from build123d import *

# Parameters (mm, degrees)
SKETCH1_W             = 80
SKETCH1_H             = 225
BOSS_EXTRUDE1_DEPTH   = 29
CUT_EXTRUDE1_REACH    = 124.871
SKETCH3_R             = 8
CUT_EXTRUDE2_DEPTH    = 20
M8_TAPPED_HOLE1_D     = 6.8
M8_TAPPED_HOLE1_DEPTH = 19.75
M8_TAPPED_HOLE1_TIP   = 2.042926105
CUT_EXTRUDE3_REACH    = 124.871
SKETCH15_W            = 12
SKETCH15_H            = 11.5
SKETCH16_R            = 8.5
CUT_EXTRUDE4_DEPTH    = 5
CUT_EXTRUDE5_REACH    = 124.871
SKETCH17_R            = 4


with BuildPart() as part:
    # Sketch1 → Boss-Extrude1 (new body)
    with BuildSketch(Plane(origin=(0, 0, 0), x_dir=(1, 0, 0), z_dir=(0, 1, 0))):
        Rectangle(SKETCH1_W, SKETCH1_H)
    extrude(amount=-BOSS_EXTRUDE1_DEPTH)

    # Sketch2 → Cut-Extrude1 (cut, up to next)
    with BuildSketch(Plane(origin=(0, 0, 0), x_dir=(1, 0, 0), z_dir=(0, 1, 0)), mode=Mode.PRIVATE) as cut_extrude1_sk1:
        with BuildLine():
            Line((30.5, 72.87), (30.5, 95.77))
            ThreePointArc((30.5, 95.77), (33, 98.27), (35.5, 95.77))
            Line((35.5, 95.77), (35.5, 72.87))
            ThreePointArc((35.5, 72.87), (33, 70.37), (30.5, 72.87))
        make_face()
    cut_extrude1_tool1 = extrude(cut_extrude1_sk1.sketch, amount=-CUT_EXTRUDE1_REACH, mode=Mode.PRIVATE) & part.part
    # Sketch2 → Cut-Extrude1 (cut, up to next)
    with BuildSketch(Plane(origin=(0, 0, 0), x_dir=(1, 0, 0), z_dir=(0, 1, 0)), mode=Mode.PRIVATE) as cut_extrude1_sk2:
        with BuildLine():
            Line((30.5, 33.86), (30.5, 48.36))
            ThreePointArc((30.5, 48.36), (33, 50.86), (35.5, 48.36))
            Line((35.5, 48.36), (35.5, 33.86))
            ThreePointArc((35.5, 33.86), (33, 31.36), (30.5, 33.86))
        make_face()
    cut_extrude1_tool2 = extrude(cut_extrude1_sk2.sketch, amount=-CUT_EXTRUDE1_REACH, mode=Mode.PRIVATE) & part.part
    # Sketch2 → Cut-Extrude1 (cut, up to next)
    with BuildSketch(Plane(origin=(0, 0, 0), x_dir=(1, 0, 0), z_dir=(0, 1, 0)), mode=Mode.PRIVATE) as cut_extrude1_sk3:
        with BuildLine():
            Line((31.5, -47.14), (31.5, -18.14))
            ThreePointArc((31.5, -18.14), (31.207106781, -17.432893219), (30.5, -17.14))
            Line((30.5, -17.14), (-7.5, -17.14))
            ThreePointArc((-7.5, -17.14), (-8.207106781, -17.432893219), (-8.5, -18.14))
            Line((-8.5, -18.14), (-8.5, -47.14))
            ThreePointArc((-8.5, -47.14), (-7.035533906, -50.675533906), (-3.5, -52.14))
            Line((-3.5, -52.14), (26.5, -52.14))
            ThreePointArc((26.5, -52.14), (30.035533906, -50.675533906), (31.5, -47.14))
        make_face()
    cut_extrude1_tool3 = extrude(cut_extrude1_sk3.sketch, amount=-CUT_EXTRUDE1_REACH, mode=Mode.PRIVATE) & part.part
    # Sketch2 → Cut-Extrude1 (cut, up to next)
    with BuildSketch(Plane(origin=(0, 0, 0), x_dir=(1, 0, 0), z_dir=(0, 1, 0)), mode=Mode.PRIVATE) as cut_extrude1_sk4:
        with BuildLine():
            Line((30.5, -95.77), (30.5, -72.87))
            ThreePointArc((30.5, -72.87), (33, -70.37), (35.5, -72.87))
            Line((35.5, -72.87), (35.5, -95.77))
            ThreePointArc((35.5, -95.77), (33, -98.27), (30.5, -95.77))
        make_face()
    cut_extrude1_tool4 = extrude(cut_extrude1_sk4.sketch, amount=-CUT_EXTRUDE1_REACH, mode=Mode.PRIVATE) & part.part
    add(cut_extrude1_tool1.solids().sort_by_distance((33, 0, -84.32))[0], mode=Mode.SUBTRACT)
    add(cut_extrude1_tool2.solids().sort_by_distance((33, 0, -41.11))[0], mode=Mode.SUBTRACT)
    add(cut_extrude1_tool3.solids().sort_by_distance((11.5, 0, 34.518764))[0], mode=Mode.SUBTRACT)
    add(cut_extrude1_tool4.solids().sort_by_distance((33, 0, 84.32))[0], mode=Mode.SUBTRACT)

    # Sketch3 → Cut-Extrude2 (cut)
    with BuildSketch(Plane(origin=(0, 0, 0), x_dir=(1, 0, 0), z_dir=(0, 1, 0))):
        with Locations(Location((15, 72.5, 0), (0, 0, 270))):
            Circle(SKETCH3_R)
        with Locations(Location((15, 41.11, 0), (0, 0, 270))):
            Circle(SKETCH3_R)
        with Locations(Location((15, -7, 0), (0, 0, 270))):
            Circle(SKETCH3_R)
        with Locations(Location((15, -72.5, 0), (0, 0, 270))):
            Circle(SKETCH3_R)
        with Locations(Location((-20, -72.5, 0), (0, 0, 270))):
            Circle(SKETCH3_R)
        with Locations(Location((-20, -7, 0), (0, 0, 270))):
            Circle(SKETCH3_R)
        with Locations(Location((-20, 41.11, 0), (0, 0, 270))):
            Circle(SKETCH3_R)
        with Locations(Location((-20, 72.5, 0), (0, 0, 270))):
            Circle(SKETCH3_R)
    extrude(amount=-CUT_EXTRUDE2_DEPTH, mode=Mode.SUBTRACT)

    # M8 Tapped Hole1
    with Locations(Plane(origin=(0, 0, 0), x_dir=(1, 0, 0), z_dir=(0, 1, 0))):
        with Locations((-25, -36), (20, 22), (-2.5, 72.5), (-2.5, -72.5)):
            Hole(M8_TAPPED_HOLE1_D / 2, depth=M8_TAPPED_HOLE1_DEPTH)
            with Locations((0, 0, -(M8_TAPPED_HOLE1_DEPTH + M8_TAPPED_HOLE1_TIP / 2))):  # 118° drill point
                Cone(0, M8_TAPPED_HOLE1_D / 2, M8_TAPPED_HOLE1_TIP, mode=Mode.SUBTRACT)

    # Sketch15 → Cut-Extrude3 (cut, up to next)
    with BuildSketch(Plane(origin=(0, 0, 0), x_dir=(1, 0, 0), z_dir=(0, 1, 0)), mode=Mode.PRIVATE) as cut_extrude3_sk1:
        with Locations((34.75, -106.75)):
            Rectangle(SKETCH15_W, SKETCH15_H)
    cut_extrude3_tool1 = extrude(cut_extrude3_sk1.sketch, amount=-CUT_EXTRUDE3_REACH, mode=Mode.PRIVATE) & part.part
    add(cut_extrude3_tool1.solids().sort_by_distance((34.75, 0, 106.75))[0], mode=Mode.SUBTRACT)

    # Sketch16 → Cut-Extrude4 (cut)
    with BuildSketch(Plane.XZ.offset(29)):
        with Locations(Location((11.5, 100, 0), (0, 0, 270))):
            Circle(SKETCH16_R)
        with Locations(Location((11.5, -100, 0), (0, 0, 270))):
            Circle(SKETCH16_R)
    extrude(amount=-CUT_EXTRUDE4_DEPTH, mode=Mode.SUBTRACT)

    # Sketch17 → Cut-Extrude5 (cut, up to next)
    with BuildSketch(Plane(origin=(0, 0, 0), x_dir=(1, 0, 0), z_dir=(0, 1, 0)), mode=Mode.PRIVATE) as cut_extrude5_sk1:
        with Locations(Location((11.5, 9.86, 0), (0, 0, 270))):
            Circle(SKETCH17_R)
    cut_extrude5_tool1 = extrude(cut_extrude5_sk1.sketch, amount=-CUT_EXTRUDE5_REACH, mode=Mode.PRIVATE) & part.part
    add(cut_extrude5_tool1.solids().sort_by_distance((11.5, 0, -9.86))[0], mode=Mode.SUBTRACT)

    # Draft1: read off the stored shape, not the designer's step
    # Draft1: loft between two sections, ruled curve by curve
    draft1_from = [
        Edge.make_three_point_arc((30.5, -24, 95.77), (31.232233047, -24, 97.537766953), (33, -24, 98.27)),
        Edge.make_three_point_arc((33, -24, 98.27), (34.767766953, -24, 97.537766953), (35.5, -24, 95.77)),
        Edge.make_three_point_arc((35.5, -24, 72.87), (34.767766953, -24, 71.102233047), (33, -24, 70.37)),
        Edge.make_three_point_arc((33, -24, 70.37), (31.232233047, -24, 71.102233047), (30.5, -24, 72.87)),
        Edge.make_line((30.5, -24, 72.87), (30.5, -24, 95.77)),
        Edge.make_line((35.5, -24, 95.77), (35.5, -24, 72.87)),
    ]
    draft1_to = [
        Edge.make_three_point_arc((29.661901532, 0, 95.77), (30.639607937, 0, 98.130392063), (33, 0, 99.108098468)),
        Edge.make_three_point_arc((33, 0, 99.108098468), (35.360392063, 0, 98.130392063), (36.338098468, 0, 95.77)),
        Edge.make_three_point_arc((36.338098468, 0, 72.87), (35.360392063, 0, 70.509607937), (33, 0, 69.531901532)),
        Edge.make_three_point_arc((33, 0, 69.531901532), (30.639607937, 0, 70.509607937), (29.661901532, 0, 72.87)),
        Edge.make_line((29.661901532, 0, 72.87), (29.661901532, 0, 95.77)),
        Edge.make_line((36.338098468, 0, 95.77), (36.338098468, 0, 72.87)),
    ]
    draft1 = Solid(Shell([*[Face.make_surface_from_curves(draft1_from[k], draft1_to[k]) for k in range(6)], Face(Wire(draft1_from)), Face(Wire(draft1_to))]))
    add(draft1, mode=Mode.SUBTRACT)

    # Draft1 2: loft between two sections, ruled curve by curve
    draft1_2_from = [
        Edge.make_three_point_arc((30.5, -24, -33.86), (31.232233047, -24, -32.092233047), (33, -24, -31.36)),
        Edge.make_three_point_arc((33, -24, -31.36), (34.767766953, -24, -32.092233047), (35.5, -24, -33.86)),
        Edge.make_three_point_arc((35.5, -24, -48.36), (34.767766953, -24, -50.127766953), (33, -24, -50.86)),
        Edge.make_three_point_arc((33, -24, -50.86), (31.232233047, -24, -50.127766953), (30.5, -24, -48.36)),
        Edge.make_line((30.5, -24, -48.36), (30.5, -24, -33.86)),
        Edge.make_line((35.5, -24, -33.86), (35.5, -24, -48.36)),
    ]
    draft1_2_to = [
        Edge.make_three_point_arc((29.661901532, 0, -33.86), (30.639607937, 0, -31.499607937), (33, 0, -30.521901532)),
        Edge.make_three_point_arc((33, 0, -30.521901532), (35.360392063, 0, -31.499607937), (36.338098468, 0, -33.86)),
        Edge.make_three_point_arc((36.338098468, 0, -48.36), (35.360392063, 0, -50.720392063), (33, 0, -51.698098468)),
        Edge.make_three_point_arc((33, 0, -51.698098468), (30.639607937, 0, -50.720392063), (29.661901532, 0, -48.36)),
        Edge.make_line((29.661901532, 0, -48.36), (29.661901532, 0, -33.86)),
        Edge.make_line((36.338098468, 0, -33.86), (36.338098468, 0, -48.36)),
    ]
    draft1_2 = Solid(Shell([*[Face.make_surface_from_curves(draft1_2_from[k], draft1_2_to[k]) for k in range(6)], Face(Wire(draft1_2_from)), Face(Wire(draft1_2_to))]))
    add(draft1_2, mode=Mode.SUBTRACT)

    # Draft1 3: loft between two sections, ruled curve by curve
    draft1_3_from = [
        Edge.make_three_point_arc((30.5, -24, -72.87), (31.232233047, -24, -71.102233047), (33, -24, -70.37)),
        Edge.make_three_point_arc((33, -24, -70.37), (34.767766953, -24, -71.102233047), (35.5, -24, -72.87)),
        Edge.make_three_point_arc((35.5, -24, -95.77), (34.767766953, -24, -97.537766953), (33, -24, -98.27)),
        Edge.make_three_point_arc((33, -24, -98.27), (31.232233047, -24, -97.537766953), (30.5, -24, -95.77)),
        Edge.make_line((30.5, -24, -95.77), (30.5, -24, -72.87)),
        Edge.make_line((35.5, -24, -72.87), (35.5, -24, -95.77)),
    ]
    draft1_3_to = [
        Edge.make_three_point_arc((29.661901532, 0, -72.87), (30.639607937, 0, -70.509607937), (33, 0, -69.531901532)),
        Edge.make_three_point_arc((33, 0, -69.531901532), (35.360392063, 0, -70.509607937), (36.338098468, 0, -72.87)),
        Edge.make_three_point_arc((36.338098468, 0, -95.77), (35.360392063, 0, -98.130392063), (33, 0, -99.108098468)),
        Edge.make_three_point_arc((33, 0, -99.108098468), (30.639607937, 0, -98.130392063), (29.661901532, 0, -95.77)),
        Edge.make_line((29.661901532, 0, -95.77), (29.661901532, 0, -72.87)),
        Edge.make_line((36.338098468, 0, -72.87), (36.338098468, 0, -95.77)),
    ]
    draft1_3 = Solid(Shell([*[Face.make_surface_from_curves(draft1_3_from[k], draft1_3_to[k]) for k in range(6)], Face(Wire(draft1_3_from)), Face(Wire(draft1_3_to))]))
    add(draft1_3, mode=Mode.SUBTRACT)

    # Draft1 4: loft between two sections, ruled curve by curve
    draft1_4_from = [
        Edge.make_three_point_arc((26.5, -24, 52.14), (30.035533906, -24, 50.675533906), (31.5, -24, 47.14)),
        Edge.make_three_point_arc((-8.5, -24, 47.14), (-7.035533906, -24, 50.675533906), (-3.5, -24, 52.14)),
        Edge.make_three_point_arc((-7.5, -24, 17.14), (-8.207106781, -24, 17.432893219), (-8.5, -24, 18.14)),
        Edge.make_three_point_arc((31.5, -24, 18.14), (31.207106781, -24, 17.432893219), (30.5, -24, 17.14)),
        Edge.make_line((-3.5, -24, 52.14), (26.5, -24, 52.14)),
        Edge.make_line((-8.5, -24, 18.14), (-8.5, -24, 47.14)),
        Edge.make_line((30.5, -24, 17.14), (-7.5, -24, 17.14)),
        Edge.make_line((31.5, -24, 47.14), (31.5, -24, 18.14)),
    ]
    draft1_4_to = [
        Edge.make_three_point_arc((26.5, 0, 52.978098468), (30.628159016, 0, 51.268159016), (32.338098468, 0, 47.14)),
        Edge.make_three_point_arc((-9.338098468, 0, 47.14), (-7.628159016, 0, 51.268159016), (-3.5, 0, 52.978098468)),
        Edge.make_three_point_arc((-7.5, 0, 16.301901532), (-8.799731891, 0, 16.840268109), (-9.338098468, 0, 18.14)),
        Edge.make_three_point_arc((32.338098468, 0, 18.14), (31.799731891, 0, 16.840268109), (30.5, 0, 16.301901532)),
        Edge.make_line((-3.5, 0, 52.978098468), (26.5, 0, 52.978098468)),
        Edge.make_line((-9.338098468, 0, 18.14), (-9.338098468, 0, 47.14)),
        Edge.make_line((30.5, 0, 16.301901532), (-7.5, 0, 16.301901532)),
        Edge.make_line((32.338098468, 0, 47.14), (32.338098468, 0, 18.14)),
    ]
    draft1_4 = Solid(Shell([*[Face.make_surface_from_curves(draft1_4_from[k], draft1_4_to[k]) for k in range(8)], Face(Wire(draft1_4_from)), Face(Wire(draft1_4_to))]))
    add(draft1_4, mode=Mode.SUBTRACT)


solid = part.part
Design review of the part built by this model. Coordinates are the model's own, in mm. A direction names the side the tool comes from. Give positions to 0.01 mm unless a question says otherwise; leave off trailing zeros. Loops run counter-clockwise (first coordinate to the right, second up) from the corner with the lowest first, then second, coordinate; pieces in that order, holes last. Notation, with made-up numbers: M 87,9 L 113,9 A17 cw 113,35 Z; hole C 0,47.25 d4. An arc over 180 degrees is marked long. One line per question, with ' | ' between items. Start each with the question number.
1. The part is to be moulded in two halves that separate along Z. For faces 4 (the face through (11.87, -26.54, -91.51)), 5 (the face through (40, -14, -4)), say which applies: released by +Z, released by -Z, zero draft, split by the parting line, or undercut.
2. Add section C-C (x = -15). Write out the cut boundary in (y, z) (3 decimals), plus the area to 3 significant figures.
3. Add section A-A (z = -9.86). Write out the cut boundary in (x, y), plus the area to 3 significant figures.
4. Add section B-B (y = -10.75). Give the number of separate pieces and of enclosed holes in the cut face, plus the area to 3 significant figures.
5. To check wall thickness, follow L1, parallel to Z at x = -23.5, y = -8.5; L2, parallel to X at y = -25.75, z = 36; L3, parallel to Z at x = -2.5, y = -6.25. State the ranges of each line that lie inside material, in increasing order.
6. Insertion check: P1, Ø8.5, axis at x = 11, z = 96, coming from the -Y side; P2, Ø8, axis at x = 14.5, z = 10, coming from the +Y side; P3, Ø1, axis at x = 31.5, z = -28.5, coming from the +Y side; P4, Ø5.5, axis at x = -2.5, z = 72.5, coming from the +Y side. Each pin has a flat end and moves straight along its axis. Give the tip position at first contact, or say it passes through.
7. For faces 1 (the face through (10.132, -9.86, -78.849)), 2 (the face through (11, -26, 52.14)), 3 (the face through (12, -24, 100)), list the 3-axis set-ups (+Z, -Z, +X, -X, +Y, -Y) from which the entire face can be reached by the end or side of a thin tool; tool diameter is ignored.
Worked out:
1) face 4: undercut | face 5: zero draft
2) outline: M -29,-112.5 L 0,-112.5 L 0,-78.745 L -20,-78.745 L -20,-66.255 L 0,-66.255 L 0,-47.355 L -20,-47.355 L -20,-34.865 L 0,-34.865 L 0,0.755 L -20,0.755 L -20,13.245 L 0,13.245 L 0,66.255 L -20,66.255 L -20,78.745 L 0,78.745 L 0,112.5 L -29,112.5 Z | area: 5,530 mm²
3) outline: M -40,-29 L 7.5,-29 L 7.5,0 L -40,0 Z; M 15.5,-29 L 40,-29 L 40,0 L 15.5,0 Z | area: 2,090 mm²
4) separate pieces: 1 | enclosed holes: 17 | area: 14,200 mm²
5) L1: z = -112.5 to -79.69, -65.31 to -48.3, -33.92 to -0.19, 14.19 to 32.95, 39.05 to 65.31, 79.69 to 112.5 | L2: x = -40 to -8.5, 31.5 to 40 | L3: z = -112.5 to -75.9, -69.1 to 16.52, 52.76 to 69.1, 75.9 to 112.5
6) P1: stops at y = -24 | P2: stops at y = -20 | P3: stops at y = 0 | P4: stops at y = -20.14
7) face 1: +Y | face 2: +Y, -Y | face 3: -Y
